Design review of the part shown in the three views and the two pictorial views. Dimensions are in mm from the part's minimum x, y and z. Coordinates: 2 decimals unless noted, no trailing zeros. Loops run counter-clockwise (first coordinate to the right, second up) from the corner with the lowest first, then second, coordinate; pieces in that order, holes last. Notation, with made-up numbers: (89.25, -28) -> (104.25, -28) arc R21 ccw to (104.25, 10) -> close; hole circle Ø2 at (35, -12). An arc over 180 degrees is marked (long way). Answer in a Markdown table with one row per item.
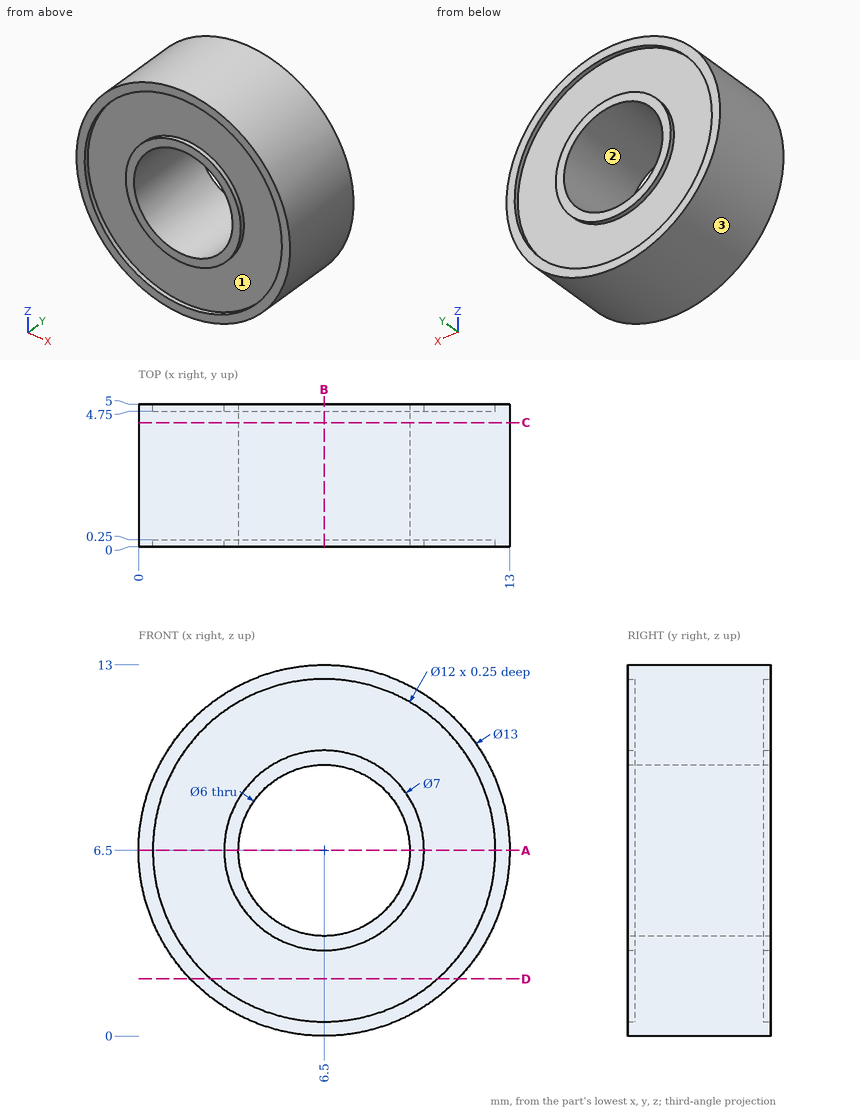
(1) To check wall thickness, follow probe 1 along X at (y, z) = (0.15, 6.5); probe 2 along X at (y, z) = (3.8, 6.5); probe 3 along Y at (x, z) = (4, 9.25). State the ranges of each line that lie inside material, in increasing order.
Evaluation:
| item | result |
|---|---|
| probe 1 | x = 0 to 0.5, 3 to 3.5, 9.5 to 10, 12.5 to 13 |
| probe 2 | x = 0 to 3.5, 9.5 to 13 |
| probe 3 | y = 0.25 to 4.75 |
(2) Draft analysis for pull direction Z (two halves, no side actions). For the marked faces 1, 2 and 3, state which applies: pulls with the +Z half, pulls with the -Z half, needs draft (parallel to the pull), parting line crosses it, or undercut.
Evaluation:
| item | result |
|---|---|
| face 1 | undercut |
| face 2 | undercut |
| face 3 | parting line crosses it |
(3) Take a section at D-D on z = 2. Give the boundary of the cut face in (x, y), and give its area (3 significant figures).
Evaluation:
| item | result |
|---|---|
| outline | (1.81, 0) -> (2.53, 0) -> (2.53, 0.25) -> (10.47, 0.25) -> (10.47, 0) -> (11.19, 0) -> (11.19, 5) -> (10.47, 5) -> (10.47, 4.75) -> (2.53, 4.75) -> (2.53, 5) -> (1.81, 5) -> close |
| area | 42.9 mm² |
(4) Take a section at B-B on x = 6.5. Give the boundary of the cut face in (y, z), and give its area (3 significant figures).
Evaluation:
| item | result |
|---|---|
| outline | (0, 0) -> (5, 0) -> (5, 0.5) -> (4.75, 0.5) -> (4.75, 3) -> (5, 3) -> (5, 3.5) -> (0, 3.5) -> (0, 3) -> (0.25, 3) -> (0.25, 0.5) -> (0, 0.5) -> close; (0, 9.5) -> (5, 9.5) -> (5, 10) -> (4.75, 10) -> (4.75, 12.5) -> (5, 12.5) -> (5, 13) -> (0, 13) -> (0, 12.5) -> (0.25, 12.5) -> (0.25, 10) -> (0, 10) -> close |
| area | 32.5 mm² |
(5) For pin 1 (3.5 mm diameter, centred on x = 6.5, z = 6.5, fed in from -Y); pin 2 (2 mm diameter, centred on y = 2, z = 9, fed in from -X); pin 3 (1.5 mm diameter, centred on x = 9.5, y = 1, fed in from -Z); pin 4 (3 mm diameter, centred on x = 3.5, y = 2.5, fed in from +Z), all flat-tipped, find the tip position at first contact; note any pin that passes through.
Evaluation:
| item | result |
|---|---|
| pin 1 | passes through |
| pin 2 | stops at x = 0.18 |
| pin 3 | stops at z = 0.4 |
| pin 4 | stops at z = 12.82 |
(6) Take a section at C-C on y = 4.35. Give the boundary of the cut face in (x, z), and give its area (3 significant figures).
Evaluation:
| item | result |
|---|---|
| outline | circle Ø13 at (6.5, 6.5); hole circle Ø6 at (6.5, 6.5) |
| area | 104 mm² |
(7) Take a section at A-A on z = 6.5. Give the boundary of the cut face in (x, y), and give its area (3 significant figures).
Evaluation:
| item | result |
|---|---|
| outline | (0, 0) -> (0.5, 0) -> (0.5, 0.25) -> (3, 0.25) -> (3, 0) -> (3.5, 0) -> (3.5, 5) -> (3, 5) -> (3, 4.75) -> (0.5, 4.75) -> (0.5, 5) -> (0, 5) -> close; (9.5, 0) -> (10, 0) -> (10, 0.25) -> (12.5, 0.25) -> (12.5, 0) -> (13, 0) -> (13, 5) -> (12.5, 5) -> (12.5, 4.75) -> (10, 4.75) -> (10, 5) -> (9.5, 5) -> close |
| area | 32.5 mm² |
